Check sheet for the modelled part. Datum: model origin and axes. Units: mm. Face numbers are marked on the shaded views. A direction names the side the tool comes from. Round coordinates to 2 decimals unless told otherwise and drop trailing zeros. Loops run counter-clockwise (first coordinate to the right, second up) from the corner with the lowest first, then second, coordinate; pieces in that order, holes last. Notation, with made-up numbers: (85.25, 16.5) -> (126.25, 16.5) arc R9 ccw to (126.25, 27.5) -> close; hole circle Ø7 at (42, 4.5). An arc over 180 degrees is marked (long way). One line per item, written item: value. Start each with the question number.
1. Material ranges on L1, parallel to Z at x = 29, y = -54.25; L2, parallel to Z at x = -8, y = -59.25, recorded low to high.
2. Release check for a two-part mould opening along X. For the marked faces 1, 2 and 3 record: +X half, -X half, draft (parallel to the pull), parting line (faces both ways), or undercut.
3. Cross-section at A-A on z = 39. Count the separate pieces of the cut face and the enclosed holes in it, then the cut area to 3 significant figures.
4. Cross-section at B-B on x = -6.5. Record the cut outline in (y, z).
5. Go/stop test with flat-tipped pins: pin 1 (5 mm diameter, centred on y = -56.5, z = 38.5, fed in from -X); pin 2 (1.5 mm diameter, centred on x = 16.5, y = -59, fed in from -Z); pin 3 (3 mm diameter, centred on y = -56, z = 23, fed in from +X); pin 4 (4 mm diameter, centred on x = 54, y = -53.5, fed in from +Z). Record where each tip stops, or that it passes through.
6. Set-up check for the marked faces 4, 5 and 6: record each of +Z, -Z, +X, -X, +Y, -Y from which the full face is reachable in a straight line by a thin tool's end or side.
from build123d import *

# Parameters (mm, degrees)
F0_W        = 120
F0_H        = 10
F1_DEPTH    = 5
F2_W        = 6
F2_H        = 10
F3_DEPTH    = 50
F4_W        = 4.6
F4_H        = 10
F5_DEPTH    = 2
F6_T1_DEPTH = 10
F6_T3_DEPTH = 22.5
F7_R        = 5
F8_R        = 0.99999


# Not quite as in the source:
# - a fillet or chamfer that OpenCascade refuses, or shapes differently, is made with other operations: its cross-section is extruded or revolved along the edge and cut away or added
# - a fillet or chamfer is up to 0.001 mm smaller than in the source, because OpenCascade refuses the exact size


with BuildPart() as f1:
    # F0 (on Top) → F1 (new body)
    with BuildSketch(Plane.XY):
        with Locations((-1.1, -55)):
            Rectangle(F0_W, F0_H)
    extrude(amount=F1_DEPTH)

    # F2 (on face) → F3 (join)
    with BuildSketch(Plane.XY.offset(5)):
        with Locations((-48.1, -55)):
            Rectangle(F2_W, F2_H)
        with Locations((-37.5, -55)):
            Rectangle(F2_W, F2_H)
        with Locations((-26.9, -55)):
            Rectangle(F2_W, F2_H)
        with Locations((-16.3, -55)):
            Rectangle(F2_W, F2_H)
        with Locations((-5.7, -55)):
            Rectangle(F2_W, F2_H)
        with Locations((4.9, -55)):
            Rectangle(F2_W, F2_H)
        with Locations((15.5, -55)):
            Rectangle(F2_W, F2_H)
        with Locations((26.1, -55)):
            Rectangle(F2_W, F2_H)
        with Locations((36.7, -55)):
            Rectangle(F2_W, F2_H)
        with Locations((47.3, -55)):
            Rectangle(F2_W, F2_H)
    extrude(amount=F3_DEPTH)

    # F4 (on face) → F5 (cut)
    with BuildSketch(Plane.XY.offset(5)):
        with Locations((-42.8, -55)):
            Rectangle(F4_W, F4_H)
        with Locations((-32.2, -55)):
            Rectangle(F4_W, F4_H)
        with Locations((-21.6, -55)):
            Rectangle(F4_W, F4_H)
        with Locations((-11, -55)):
            Rectangle(F4_W, F4_H)
        with Locations((-0.4, -55)):
            Rectangle(F4_W, F4_H)
        with Locations((10.2, -55)):
            Rectangle(F4_W, F4_H)
        with Locations((20.8, -55)):
            Rectangle(F4_W, F4_H)
        with Locations((31.4, -55)):
            Rectangle(F4_W, F4_H)
        with Locations((42, -55)):
            Rectangle(F4_W, F4_H)
    extrude(amount=-F5_DEPTH, mode=Mode.SUBTRACT)

    # F6: fillet of radius 2.5 on 22 edges, made by hand

    # F6_s2 → F6_t1 (join)
    with BuildSketch(Plane.XZ.offset(50)):
        with BuildLine():
            ThreePointArc((-45.1, 5.5), (-44.367766953, 3.732233047), (-42.6, 3))
            Line((-42.6, 3), (-45.1, 3))
            Line((-45.1, 3), (-45.1, 5.5))
        make_face()
        with BuildLine():
            ThreePointArc((-43, 3), (-41.232233047, 3.732233047), (-40.5, 5.5))
            Line((-40.5, 5.5), (-40.5, 3))
            Line((-40.5, 3), (-43, 3))
        make_face()
        with BuildLine():
            ThreePointArc((-32.4, 3), (-30.632233047, 3.732233047), (-29.9, 5.5))
            Line((-29.9, 5.5), (-29.9, 3))
            Line((-29.9, 3), (-32.4, 3))
        make_face()
        with BuildLine():
            ThreePointArc((-23.9, 5.5), (-23.167766953, 3.732233047), (-21.4, 3))
            Line((-21.4, 3), (-23.9, 3))
            Line((-23.9, 3), (-23.9, 5.5))
        make_face()
        with BuildLine():
            ThreePointArc((-21.8, 3), (-20.032233047, 3.732233047), (-19.3, 5.5))
            Line((-19.3, 5.5), (-19.3, 3))
            Line((-19.3, 3), (-21.8, 3))
        make_face()
        with BuildLine():
            ThreePointArc((-13.3, 5.5), (-12.567766953, 3.732233047), (-10.8, 3))
            Line((-10.8, 3), (-13.3, 3))
            Line((-13.3, 3), (-13.3, 5.5))
        make_face()
        with BuildLine():
            ThreePointArc((-11.2, 3), (-9.432233047, 3.732233047), (-8.7, 5.5))
            Line((-8.7, 5.5), (-8.7, 3))
            Line((-8.7, 3), (-11.2, 3))
        make_face()
        with BuildLine():
            ThreePointArc((-2.7, 5.5), (-1.967766953, 3.732233047), (-0.2, 3))
            Line((-0.2, 3), (-2.7, 3))
            Line((-2.7, 3), (-2.7, 5.5))
        make_face()
        with BuildLine():
            ThreePointArc((-0.6, 3), (1.167766953, 3.732233047), (1.9, 5.5))
            Line((1.9, 5.5), (1.9, 3))
            Line((1.9, 3), (-0.6, 3))
        make_face()
        with BuildLine():
            ThreePointArc((10, 3), (11.767766953, 3.732233047), (12.5, 5.5))
            Line((12.5, 5.5), (12.5, 3))
            Line((12.5, 3), (10, 3))
        make_face()
        with BuildLine():
            ThreePointArc((20.6, 3), (22.367766953, 3.732233047), (23.1, 5.5))
            Line((23.1, 5.5), (23.1, 3))
            Line((23.1, 3), (20.6, 3))
        make_face()
        with BuildLine():
            ThreePointArc((31.2, 3), (32.967766953, 3.732233047), (33.7, 5.5))
            Line((33.7, 5.5), (33.7, 3))
            Line((33.7, 3), (31.2, 3))
        make_face()
        with BuildLine():
            ThreePointArc((41.8, 3), (43.567766953, 3.732233047), (44.3, 5.5))
            Line((44.3, 5.5), (44.3, 3))
            Line((44.3, 3), (41.8, 3))
        make_face()
        with BuildLine():
            ThreePointArc((39.7, 5.5), (40.432233047, 3.732233047), (42.2, 3))
            Line((42.2, 3), (39.7, 3))
            Line((39.7, 3), (39.7, 5.5))
        make_face()
        with BuildLine():
            ThreePointArc((29.1, 5.5), (29.832233047, 3.732233047), (31.6, 3))
            Line((31.6, 3), (29.1, 3))
            Line((29.1, 3), (29.1, 5.5))
        make_face()
        with BuildLine():
            ThreePointArc((18.5, 5.5), (19.232233047, 3.732233047), (21, 3))
            Line((21, 3), (18.5, 3))
            Line((18.5, 3), (18.5, 5.5))
        make_face()
        with BuildLine():
            ThreePointArc((7.9, 5.5), (8.632233047, 3.732233047), (10.4, 3))
            Line((10.4, 3), (7.9, 3))
            Line((7.9, 3), (7.9, 5.5))
        make_face()
        with BuildLine():
            ThreePointArc((50.3, 7.5), (51.032233047, 5.732233047), (52.8, 5))
            Line((52.8, 5), (50.3, 5))
            Line((50.3, 5), (50.3, 7.5))
        make_face()
        with BuildLine():
            ThreePointArc((-53.6, 5), (-51.832233047, 5.732233047), (-51.1, 7.5))
            Line((-51.1, 7.5), (-51.1, 5))
            Line((-51.1, 5), (-53.6, 5))
        make_face()
        with BuildLine():
            ThreePointArc((-34.5, 5.5), (-33.767766953, 3.732233047), (-32, 3))
            Line((-32, 3), (-34.5, 3))
            Line((-34.5, 3), (-34.5, 5.5))
        make_face()
    extrude(amount=F6_T1_DEPTH)

    # F6_s4 → F6_t3 (cut)
    with BuildSketch(Plane.XZ.offset(43.75)):
        with BuildLine():
            ThreePointArc((58.9, 2.5), (58.167766953, 4.267766953), (56.4, 5))
            Line((56.4, 5), (58.9, 5))
            Line((58.9, 5), (58.9, 2.5))
        make_face()
        with BuildLine():
            ThreePointArc((-58.6, 5), (-60.367766953, 4.267766953), (-61.1, 2.5))
            Line((-61.1, 2.5), (-61.1, 5))
            Line((-61.1, 5), (-58.6, 5))
        make_face()
    extrude(amount=F6_T3_DEPTH, mode=Mode.SUBTRACT)

    # F7
    f7_edges = [f1.edges().sort_by_distance(p)[0] for p in [
        (-51.1, -55, 55),
        (-40.5, -55, 55),
        (-29.9, -55, 55),
        (-19.3, -55, 55),
        (-8.7, -55, 55),
        (1.9, -55, 55),
        (12.5, -55, 55),
        (23.1, -55, 55),
        (33.7, -55, 55),
        (44.3, -55, 55),
    ]]
    fillet(f7_edges, radius=F7_R)

    # F8 (radius 1 in the source; OpenCascade refuses exactly that, so slightly less here)
    f8_edges = [f1.edges().sort_by_distance(p)[0] for p in [
        (-45.1, -55, 55),
        (-34.5, -55, 55),
        (-23.9, -55, 55),
        (-13.3, -55, 55),
        (-2.7, -55, 55),
        (7.9, -55, 55),
        (18.5, -55, 55),
        (29.1, -55, 55),
        (39.7, -55, 55),
        (50.3, -55, 55),
    ]]
    fillet(f8_edges, radius=F8_R)


solid = f1.part
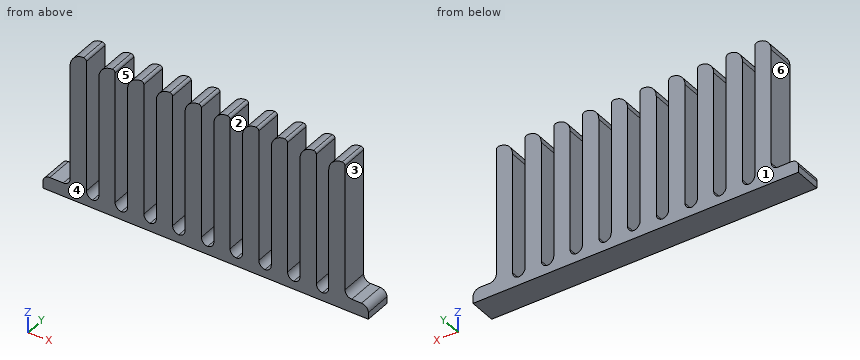
Taken from the geometry:
1. L1: z = 0 to 54.44
1. L2: z = 0 to 52.55
2. face 1: draft
2. face 2: undercut
2. face 3: +X half
3. separate pieces: 10
3. enclosed holes: 0
3. area: 600 mm2
4. outline: (-60, 0) -> (-50, 0) -> (-50, 54.14) -> (-60, 54.14) -> close
5. pin 1: stops at x = -51.1
5. pin 2: stops at z = 0
5. pin 3: stops at x = 50.3
5. pin 4: stops at z = 5.13
6. face 4: +Z, -Z, +X, -X, -Y
6. face 5: +Z, +Y, -Y
6. face 6: +Z, -X, +Y, -Y
